Autodesk Inventor part; units mm, degrees
ref_plane "YZ Plane" through (0, 0, 0) normal (1, 0, 0) x (0, 1, 0)
ref_plane "XZ Plane" through (0, 0, 0) normal (0, 1, 0) x (-1, 0, 0)
ref_plane "XY Plane" through (0, 0, 0) normal (0, 0, 1) x (1, 0, 0)
sketch "Sketch1" plane through (0, 0, 0) normal (0, 1, 0) x (-1, 0, 0)
  line L0 (0, 0) -> (9.5, 0)
  line L1 (9.5, 0) -> (9.5, -64)
  line L2 (9.5, -64) -> (0, -64)
  line L3 (0, -64) -> (0, 0)
  circle A0 centre (3.7, -11.5) radius 2.25
  circle A1 centre (3.7, -59.5) radius 2.25
  line L4 (3.7, -11.5) -> (3.7, -59.5) construction
  dimension "d1" = 9.5
  dimension "d2" = 64
  dimension "d3" = 4.5
  dimension "d4" = 48
  dimension "d6" = 3.7
  dimension "d17" = 4.5
extrude "Extrusion1" add sketch "Sketch1" along normal blind 12
sketch "Sketch2" plane through (-9.5, 0, 0) normal (0, 0, 1) x (1, 0, 0)
  line L0 (9.5, 12) -> (0, 12)
  line L1 (3, 12) -> (8.4, 12)
  line L2 (8.4, 12) -> (8.4, 10.8)
  line L3 (8.4, 10.8) -> (3, 10.8)
  line L4 (3, 10.8) -> (3, 12)
  line L5 (9.5, 0) -> (9.5, 12)
  line L6 (3.55, 0) -> (8.05, 0)
  line L7 (3.55, 12) -> (8.05, 12)
  line L8 (9.5, 0) -> (9.5, 12)
  line L9 (9.5, 0) -> (9.5, 12)
  line L10 (3.55, 12) -> (8.05, 12)
  line L11 (3.55, 12) -> (3.55, 0)
  line L12 (3.55, 12) -> (8.05, 12)
  line L13 (3.55, 0) -> (8.05, 0)
  line L14 (3.55, 12) -> (8.05, 12)
  line L15 (3.55, 0) -> (8.05, 0)
  line L16 (3.55, 12) -> (8.05, 12)
  line L17 (3.55, 0) -> (8.05, 0)
  dimension "d9" = 1.1
  dimension "d10" = 5.4
  dimension "d11" = 1.2
  dimension "d76" = 12
extrude "Extrusion2" cut sketch "Sketch2" against normal up to next
sketch "Sketch3" plane through (0, 0, 0) normal (0, -1, 0) x (1, 0, 0)
  circle A0 centre (-3.7, -11.5) radius 2.25
  circle A1 centre (-3.7, -11.5) radius 3.75
  circle A2 centre (-3.7, -59.5) radius 2.25
  circle A3 centre (-3.7, -59.5) radius 3.75
  point P0 (0, 0)
  dimension "d14" = 7.5
extrude "Extrusion3" cut sketch "Sketch3" against normal blind 3
fillet "Fillet1" radius 1 4 edges at (0, 1.5, -58.8897) (0, 1.5, -60.1103) (0, 1.5, -10.8897) (0, 1.5, -12.1103)
fillet "Fillet2" radius 4 2 edges at (-9.5, 6, -64) (-9.5, 6, 0)
sketch "Sketch28" plane through (0, 0, 0) normal (0, -1, 0) x (1, 0, 0)
  arc A0 (-1.5684, -56.4147) -> (0, -55.592) centre (-1, -55.592) ccw
  line L0 (0, -55.592) -> (0, -53)
  line L1 (0, -15.408) -> (0, -55.592)
  line L2 (-9.5, -60) -> (-9.5, -4)
  line L3 (0, -53) -> (-9.5, -53)
  line L4 (-9.5, -53) -> (-9.5, -34)
  line L5 (-9.5, -34) -> (0, -34)
  line L6 (0, -34) -> (0, -53)
  point P0 (0, 0)
  point P1 (0, -34)
  dimension "d107" = 2.592
  dimension "d108" = 19
extrude "Extrusion19" add sketch "Sketch28" along normal blind 20
sketch "Sketch40" plane through (0, -20, 0) normal (0, -1, 0) x (1, 0, 0)
  line L0 (0, -53) -> (-9.5, -53)
  line L1 (-9.5, -53) -> (-9.5, -73)
  line L2 (-9.5, -73) -> (0, -73)
  line L3 (0, -73) -> (0, -43)
  line L4 (0, 0) -> (0, -64)
  line L5 (0, -43) -> (-9.5, -43)
  line L6 (-9.5, -43) -> (-9.5, -53)
  line L7 (-9.5, -43) -> (0, -43)
  line L8 (0, -43) -> (0, -73)
  line L9 (0, -73) -> (-9.5, -73)
  line L10 (-9.5, -73) -> (-9.5, -43)
  dimension "d130" = 20
  dimension "d131" = 30
extrude "Extrusion21" add sketch "Sketch40" along normal blind 10
sketch "Sketch41" plane through (0, 0, -53) normal (0, 0, -1) x (-1, 0, 0)
  point P0 (0, 0)
sketch "Sketch42" plane through (0, -30, 0) normal (0, -1, 0) x (1, 0, 0)
  line L0 (0, -73) -> (0, -53)
  line L1 (0, -73) -> (30, -73)
  line L2 (30, -73) -> (30, -66)
  line L3 (30, -66) -> (-20, -66)
  line L4 (-20, -66) -> (-20, -73)
  line L5 (-20, -73) -> (0, -73)
  point P0 (0, 0)
  dimension "d134" = 30
  dimension "d135" = 7
  dimension "d137" = 50
extrude "Extrusion22" add sketch "Sketch42" along normal blind 7
sketch "Sketch44" plane through (0, -37, 0) normal (0, -1, 0) x (1, 0, 0)
  line L0 (-20, -73) -> (30, -73)
  line L1 (30, -66) -> (-20, -66)
  line L2 (-20, -73) -> (30, -73)
  line L3 (30, -73) -> (30, -66)
  line L4 (30, -66) -> (-20, -66)
  line L5 (-20, -66) -> (-20, -73)
  point P0 (0, 0)
sketch "Sketch45" plane through (-20, -30, -73) normal (-1, 0, 0) x (0, 0, 1)
  line L0 (7, 0) -> (7, -7)
  arc A0 (7, -7) -> (7, -57) centre (31.4949, -32) ccw
  point P0 (73, 30)
  dimension "d142" = 50
  dimension "d143" = 35
sweep "Sweep3" add profiles "Sketch44" path "Sketch45"
sketch "Sketch46" plane through (-20, -87, -66) normal (0, -0.6998542, 0.7142857) x (1, 0, 0)
  line L0 (0, 35.7143) -> (0, 0)
  line L1 (0, 0) -> (25, -10.3821) construction
  line L2 (50, 0) -> (0, 0)
  line L3 (25, -10.3821) -> (50, 0) construction
  spline S0 degree 2 poles (0, 0) (25, -10.3821) (50, 0) knots 1 1 1 2 2 2
  line L4 (0, 0) -> (50, 0)
  line L5 (60.7, 35) -> (-10.7, 35)
  point P0 (20, 108.3332)
revolve "Revolution1" cut sketch "Sketch46" angle 90 about axis through (5, -62, -41.5051) along (1, 0, 0)
sketch "Sketch47" plane through (-20, -92, -70.899) normal (0, -0.6998542, 0.7142857) x (1, 0, 0)
  point P0 (20, 115.3332)
properties part number "Back"
Work out the finished part from the listing and answer in its coordinate system (mm). A direction names the side the tool comes from. Give positions to 0.01 mm unless a question says otherwise; leave off trailing zeros. Write each loop counter-clockwise with the first axis right and the second up, starting at its lowest first coordinate (ties: lowest second). Pieces come first, ordered by that corner, then holes.
(1) The mould has two halves that part along Z. Classify faces 5 (the flat face through (4.88, -36.04, -68)), 6 (the flat face through (4.7, -30.2, -73)), 7 (the flat face through (-5, -25, -43)): pulls with the +Z half, pulls with the -Z half, needs draft (parallel to the pull), parting line crosses it, or undercut.
Final values:
face 5: undercut
face 6: pulls with the -Z half
face 7: pulls with the +Z half
(2) Which of the six approach directions +Z, -Z, +X, -X, +Y, -Y give full straight-line access (tool end or side, diameter ignored) to faces 1 (the flat face through (-4, 10.8, -32)), 2 (the flat face through (-5, -30, -54)), 3 (the flat face through (-7, 0, -57)), 4 (the cylindrical face through (-7.45, 1.48, -11.39))?
Final values:
face 1: +Z, -Z, +Y
face 2: +Z, +X, -X, -Y
face 3: -Z, +X, -X
face 4: -Y
(3) Straight lines are drawn through the part: line 1 (Z direction, x = -3.7, y = 1.1); line 2 (Z direction, x = -3.7, y = 6); line 3 (X direction, y = 9, z = -59.5). For each, find the intervals that lie inside material, in ascending order.
Final values:
line 1: z = -64 to -63.25, -55.75 to -15.25, -7.75 to 0
line 2: z = -64 to -61.75, -57.25 to -13.75, -9.25 to 0
line 3: x = -9.5 to -5.95, -1.45 to 0
(4) Flat-ended cylindrical pins translate along their axes: pin 1 Ø12.5 at (y, z) = (-17, -35.5) entering from +X; pin 2 Ø5 at (x, y) = (-3.5, -26.5) entering from +Z; pin 3 Ø2 at (y, z) = (-10.5, -47) entering from -X; pin 4 Ø4.5 at (x, z) = (-3, -36.5) entering from +Y. Find the tip coordinate at first contact, or state that the pin passes through.
Final values:
pin 1: stops at x = 0
pin 2: stops at z = -43
pin 3: stops at x = -9.5
pin 4: stops at y = 12
(5) The part is cut by section A-A on z = -11.5. Write down the section's boundary in (x, y).
Final values:
outline: (-9.5, 0) - (-7.45, 0) - (-7.45, 3) - (-5.95, 3) - (-5.95, 10.8) - (-6.5, 10.8) - (-6.5, 12) - (-9.5, 12) - close; (-1.45, 3) - (0, 3) - (0, 12) - (-1.1, 12) - (-1.1, 10.8) - (-1.45, 10.8) - close
(6) The part is cut by section C-C on x = -3.7. Count the separate pieces of the cut face and the enclosed holes in it, plus the area to 3 significant figures.
Final values:
separate pieces: 3
enclosed holes: 0
area: 1,450 mm2
(7) The part is cut by section B-B on y = -18.5. Write down the section's boundary in (x, z), plus the area to 4 significant figures.
Final values:
outline: (-9.5, -53) - (0, -53) - (0, -34) - (-9.5, -34) - close
area: 180.5 mm2
